Input: part model. Units: mm. Frame: model coordinates. Face numbers are marked on the shaded views. A direction names the side the tool comes from. Give positions to 0.01 mm unless a question says otherwise; leave off trailing zeros. Loops run counter-clockwise (first coordinate to the right, second up) from the corner with the lowest first, then second, coordinate; pieces in that order, holes last. Notation, with made-up numbers: M 69.5,25.5 L 107.5,25.5 A22 ccw 107.5,31.5 Z; hole C -0.75,-37.75 d10. An arc over 180 degrees is marked long. One line per item, written item: value. Start each with the question number.
(1) Pin query (flat end, axial travel): P1, Ø1.6, axis at y = 3, z = 5.5, coming from the +X side; P2, Ø3.5, axis at y = 2.5, z = 5.5, coming from the -X side; P3, Ø0.8, axis at x = 10, y = 3.5, coming from the +Z side. Return the tip coordinate at first contact, or that it passes through.
(2) Ray query, line 1 along X through (y, z) = (2, 0) (3 decimals); line 2 along X through (y, z) = (2, 3.5); line 3 along Z through (x, y) = (9.5, 3) (3 decimals). Return the intervals inside material, ascending. Write a range as from..to.
(3) Section C-C on y = 0.5. Output: boundary loops of the cut face in (x, z) (3 decimals).
(4) Section A-A on x = 9.5. Output: boundary loops of the cut face in (y, z) (3 decimals), plus the area to 3 significant figures.
(5) Section B-B on z = 3.25. Output: boundary loops of the cut face in (x, y), plus the area to 3 significant figures.
(6) Section D-D on z = 0. Output: boundary loops of the cut face in (x, y) (3 decimals).
(7) Access query for the marked faces 1 and 2. Directions: +Z, -Z, +X, -X, +Y, -Y. A direction counts if a zero-diameter tool reaches every point of the face in a straight line with its end or side. Return the directions, or none.
(8) Pull-direction query (Z, two-part tool) for the marked faces 3, 4, 5 and 6; classes: released by +Z, released by -Z, zero draft, split by the parting line, or undercut.
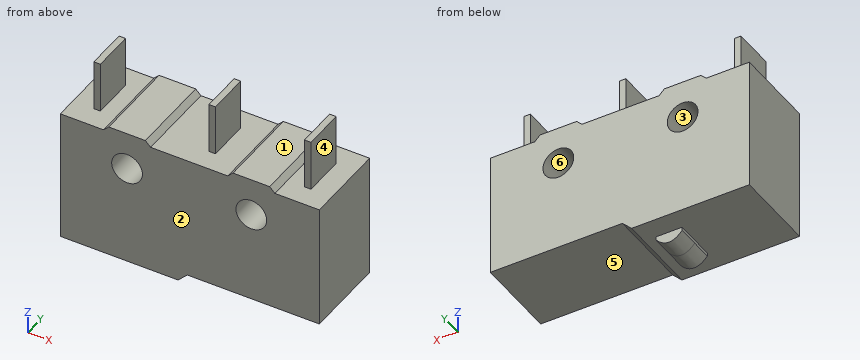
```python
from build123d import *

# Parameters (mm, degrees)
SKETCH2_R                = 1.175
BOSS_EXTRUDE1_DEPTH      = 6.4
BOSS_EXTRUDE2_DEPTH      = 1.6
BOSS_EXTRUDE2_DEPTH_BACK = 1.6
SKETCH4_W                = 0.5
SKETCH4_H                = 3.9
BOSS_EXTRUDE3_DEPTH      = 1.6
BOSS_EXTRUDE3_DEPTH_BACK = 1.6


with BuildPart() as part:
    # Sketch2 → Boss-Extrude1 (new body)
    with BuildSketch(Plane(origin=(0, 0, 0), x_dir=(1, 0, 0), z_dir=(0, 1, 0))):
        Polygon((0, -2.9), (-1.4, -2.9), (-1.8, -2.5), (-5.1, -2.5), (-5.1, 7.7), (3.9, 7.7), (4.6, 7), (14.7, 7), (14.7, -2.5), (11.3, -2.5), (10.9, -2.9), (9.5, -2.9), (8.1, -2.9), (7.7, -2.5), (1.8, -2.5), (1.4, -2.9), align=None)
        Circle(SKETCH2_R, mode=Mode.SUBTRACT)
        with Locations((9.5, 0)):
            Circle(SKETCH2_R, mode=Mode.SUBTRACT)
    extrude(amount=BOSS_EXTRUDE1_DEPTH)

    # Sketch3 → Boss-Extrude2 (add, two sides)
    with BuildSketch(Plane(origin=(0, 3.2, 0), x_dir=(1, 0, 0), z_dir=(0, 1, 0))) as boss_extrude2_sk:
        with BuildLine():
            Line((3, 7.7), (1, 7.7))
            Line((1, 7.7), (1, 7.954))
            add(Edge.make_bspline(
                [(1, 7.954), (2, 9.1224), (3, 7.954)],
                knots=[0, 0, 0, 1, 1, 1], degree=2))
            Line((3, 7.954), (3, 7.7))
        make_face()
    extrude(amount=BOSS_EXTRUDE2_DEPTH)
    extrude(boss_extrude2_sk.sketch, amount=-BOSS_EXTRUDE2_DEPTH_BACK)

    # Sketch4 → Boss-Extrude3 (add, two sides)
    with BuildSketch(Plane(origin=(0, 3.2, 0), x_dir=(1, 0, 0), z_dir=(0, 1, 0))) as boss_extrude3_sk:
        with Locations((-3.25, -4.45)):
            Rectangle(SKETCH4_W, SKETCH4_H)
        with Locations((5.55, -4.45)):
            Rectangle(SKETCH4_W, SKETCH4_H)
        with Locations((12.85, -4.45)):
            Rectangle(SKETCH4_W, SKETCH4_H)
    extrude(amount=BOSS_EXTRUDE3_DEPTH)
    extrude(boss_extrude3_sk.sketch, amount=-BOSS_EXTRUDE3_DEPTH_BACK)


solid = part.part
```
Output values:
1. P1: stops at x = 13.1
1. P2: stops at x = -3.5
1. P3: stops at z = 2.9
2. line 1: x = -5.1..-1.175, 1.175..8.325, 10.675..14.7
2. line 2: x = -3.5..-3, 5.3..5.8, 12.6..13.1
2. line 3: z = -7..-1.175, 1.175..2.9
3. outline: M -5.1,-7.7 L 3.9,-7.7 L 4.6,-7 L 14.7,-7 L 14.7,2.5 L 11.3,2.5 L 10.9,2.9 L 8.1,2.9 L 7.7,2.5 L 1.8,2.5 L 1.4,2.9 L -1.4,2.9 L -1.8,2.5 L -5.1,2.5 Z; hole C 0,0 d2.35; hole C 9.5,0 d2.35
4. outline: M 0,-7 L 6.4,-7 L 6.4,-1.175 L 0,-1.175 Z; M 0,1.175 L 6.4,1.175 L 6.4,2.9 L 0,2.9 Z
4. area: 48.3 mm²
5. outline: M -3.5,1.6 L -3,1.6 L -3,4.8 L -3.5,4.8 Z; M 5.3,1.6 L 5.8,1.6 L 5.8,4.8 L 5.3,4.8 Z; M 12.6,1.6 L 13.1,1.6 L 13.1,4.8 L 12.6,4.8 Z
5. area: 4.80 mm²
6. outline: M -5.1,0 L -1.175,0 L -1.175,6.4 L -5.1,6.4 Z; M 1.175,0 L 8.325,0 L 8.325,6.4 L 1.175,6.4 Z; M 10.675,0 L 14.7,0 L 14.7,6.4 L 10.675,6.4 Z
7. face 1: +Z, +Y, -Y
7. face 2: +Z, -Z, +X, -X, -Y
8. face 3: undercut
8. face 4: zero draft
8. face 5: released by -Z
8. face 6: undercut
